Verification items for the finished model (mm, model axes). Give positions to 0.01 mm unless a question says otherwise; leave off trailing zeros. Loops run counter-clockwise (first coordinate to the right, second up) from the corner with the lowest first, then second, coordinate; pieces in that order, holes last. Notation, with made-up numbers: M 59,-5.75 L 100,-5.75 A24 cw 100,24.25 Z; hole C -8.5,63.25 d7. An arc over 180 degrees is marked long. Answer in a Markdown table with one row per item.
```python
from build123d import *

# Parameters (mm, degrees)
SKETCH4_R         = 0.4
SKETCH5_R         = 0.7
CIRPATTERN2_COUNT = 2
CIRPATTERN2_ANGLE = 90


# Read off the part's stored shape, not the designer's step: CirPattern1
with BuildPart() as part:
    # Sweep1: sweep along a path in Sketch2
    with BuildLine(Plane(origin=(0, 0, 0), x_dir=(1, 0, 0), z_dir=(0, 1, 0))) as sweep1_path:
        Line((0, 0), (0, -10))
    # Sketch4 → Sweep1 (sweep)
    with BuildSketch(Plane.XY):
        Circle(SKETCH4_R)
    sweep1 = sweep(path=sweep1_path.line)

    # Sketch5 → Loft1 section 0
    with BuildSketch(Plane.XY.offset(10), mode=Mode.PRIVATE) as loft1_s0:
        Circle(SKETCH5_R)
    loft1 = loft([loft1_s0.sketch, Vertex(0, 0, 11.5)])

    # CirPattern1 outline → CirPattern1 (revolve)
    with BuildSketch(Plane.YX):
        Polygon((0.7, 10), (0, 11.5), (0, 0), (0.4, 0), (0.4, 10), align=None)
    revolve(axis=Axis((0, 0, 0), (1, 0, 0)))

    # CirPattern2: Sweep1, Loft1 ×2 about axis
    cirpattern2_axis = Axis((0, 0, 0), (-1, 0, 0))
    add([sweep1.rotate(cirpattern2_axis, i * CIRPATTERN2_ANGLE / (CIRPATTERN2_COUNT - 1)) for i in range(1, CIRPATTERN2_COUNT)])
    add([loft1.rotate(cirpattern2_axis, i * CIRPATTERN2_ANGLE / (CIRPATTERN2_COUNT - 1)) for i in range(1, CIRPATTERN2_COUNT)])


solid = part.part
```
Item 1: Scan line: L1, parallel to Y at x = 8, z = 0. Record every from-to range of solid material in increasing order. Write a range as [from, to].
Reported:
| item | result |
|---|---|
| L1 | y = [-0.4, 0.4] |
Item 2: Sectioned sample at A-A (y = 4.5). Record the cut outline in (x, z).
Reported:
| item | result |
|---|---|
| outline | C 0,0 d0.8 |
Item 3: Go/stop test with flat-tipped pins: pin 1 (5 mm diameter, centred on x = 1.5, y = 6.5, fed in from +Z); pin 2 (0.7 mm diameter, centred on y = 0, z = -0.5, fed in from -X); pin 3 (1.1 mm diameter, centred on x = -0.5, y = 0, fed in from -Z). Record where each tip stops, or that it passes through.
Reported:
| item | result |
|---|---|
| pin 1 | stops at z = 0.4 |
| pin 2 | stops at x = -0.37 |
| pin 3 | stops at z = -0.4 |
Item 4: Release check for a two-part mould opening along Y. For faces 1 (the conical face through (0.255, 10.927, -0.08)), 2 (the conical face through (-0.06, -0.26, 10.93)), 3 (the cylindrical face through (-0.32, 5.07, 0.24)) record: released by +Y, released by -Y, zero draft, split by the parting line, or undercut.
Reported:
| item | result |
|---|---|
| face 1 | released by +Y |
| face 2 | split by the parting line |
| face 3 | undercut |
